from build123d import *

# Parameters (mm, degrees)
MODEL_W             = 6
MODEL_H             = 6
BOSS_EXTRUDE1_DEPTH = 6


with BuildPart() as part:
    # Model → Boss-Extrude1 (new body)
    with BuildSketch(Plane.XY):
        with BuildLine():
            Line((3491.847275697, 1193.017146611), (3491.847275697, 1187.017146611))
            Line((3491.847275697, 1187.017146611), (3485.847275697, 1187.017146611))
            Line((3485.847275697, 1187.017146611), (3485.847275697, 1193.017146611))
            Line((3485.847275697, 1193.017146611), (3474.204418554, 1193.017146611))
            ThreePointArc((3474.204418554, 1193.017146611), (3501.847275697, 1220.660003754), (3529.49013284, 1193.017146611))
            Line((3529.49013284, 1193.017146611), (3491.847275697, 1193.017146611))
        make_face()
        with Locations((3514.847275697, 1206.017146611)):
            Rectangle(MODEL_W, MODEL_H, mode=Mode.SUBTRACT)
        with Locations((3488.847275697, 1206.017146611)):
            Rectangle(MODEL_W, MODEL_H, mode=Mode.SUBTRACT)
        with Locations((3501.847275697, 1212.017146611)):
            Rectangle(MODEL_W, MODEL_H, mode=Mode.SUBTRACT)
        with Locations((3501.847275697, 1199.841605445)):
            Rectangle(MODEL_W, MODEL_H, mode=Mode.SUBTRACT)
    extrude(amount=BOSS_EXTRUDE1_DEPTH)


solid = part.part
Model file for the job. Use its own axes, mm. A direction names the side the tool comes from. Give positions to 0.01 mm unless a question says otherwise; leave off trailing zeros. Loops run counter-clockwise (first coordinate to the right, second up) from the corner with the lowest first, then second, coordinate; pieces in that order, holes last.
1) Wall check: line 1 (Y direction, x = 3502.5, z = 5.2); line 2 (Y direction, x = 3502, z = 4.2); line 3 (X direction, y = 1205, z = 3.8). Give the ranges that are in metal, low to high.
2) Saw through at A-A (z = 1). Write the cut outline in (x, y), plus the area to 3 significant figures.
3) Saw through at D-D (x = 3516.5). Write the cut outline in (y, z).
4) Flat gauge pins, fed straight in: pin 1 Ø3 at (y, z) = (1204.5, 2.5) entering from -X; pin 2 Ø3 at (x, z) = (3488.5, 4.5) entering from +Y; pin 3 Ø1.8 at (x, z) = (3515.5, 2) entering from -Y. Where does each tip first touch, or does it go through?
5) Pull direction Y, two halves, no side cores. Call faces 5 (the flat face through (3491.847, 1190, 3)), 6 (the flat face through (3504.847, 1212, 3)), 7 (the flat face through (3480, 1193.017, 3)): +Y half, -Y half, draft (parallel to the pull), parting line (faces both ways), or undercut.
6) Saw through at B-B (y = 1200). Write the cut outline in (x, z).
7) Tool access for faces 1 (the flat face through (3485.847, 1190, 3)), 2 (the flat face through (3502, 1204, 6)), 3 (the flat face through (3511, 1193.017, 3)), 4 (the flat face through (3511.847, 1206, 3)): list every direction of +Z, -Z, +X, -X, +Y, -Y with a clear straight run to the whole face (end or side of a thin tool).
8) Saw through at C-C (y = 1204). Write the cut outline in (x, z), plus the area to 3 significant figures.
Answer block:
1. line 1: y = 1193.02 to 1196.84, 1202.84 to 1209.02, 1215.02 to 1220.65
1. line 2: y = 1193.02 to 1196.84, 1202.84 to 1209.02, 1215.02 to 1220.66
1. line 3: x = 3476.94 to 3485.85, 3491.85 to 3511.85, 3517.85 to 3526.76
2. outline: (3474.2, 1193.02) - (3485.85, 1193.02) - (3485.85, 1187.02) - (3491.85, 1187.02) - (3491.85, 1193.02) - (3529.49, 1193.02) arc R27.64 ccw to start; hole (3485.85, 1203.02) - (3491.85, 1203.02) - (3491.85, 1209.02) - (3485.85, 1209.02) - close; hole (3498.85, 1196.84) - (3504.85, 1196.84) - (3504.85, 1202.84) - (3498.85, 1202.84) - close; hole (3498.85, 1209.02) - (3504.85, 1209.02) - (3504.85, 1215.02) - (3498.85, 1215.02) - close; hole (3511.85, 1203.02) - (3517.85, 1203.02) - (3517.85, 1209.02) - (3511.85, 1209.02) - close
2. area: 1,090 mm2
3. outline: (1193.02, 0) - (1203.02, 0) - (1203.02, 6) - (1193.02, 6) - close; (1209.02, 0) - (1216.46, 0) - (1216.46, 6) - (1209.02, 6) - close
4. pin 1: stops at x = 3476.07
4. pin 2: stops at y = 1217.99
4. pin 3: stops at y = 1193.02
5. face 5: draft
5. face 6: undercut
5. face 7: -Y half
6. outline: (3475.1, 0) - (3498.85, 0) - (3498.85, 6) - (3475.1, 6) - close; (3504.85, 0) - (3528.59, 0) - (3528.59, 6) - (3504.85, 6) - close
7. face 1: +Z, -Z, -X, -Y
7. face 2: +Z, +X, -X, +Y, -Y
7. face 3: +Z, -Z, +X, -Y
7. face 4: +Z, -Z
8. outline: (3476.48, 0) - (3485.85, 0) - (3485.85, 6) - (3476.48, 6) - close; (3491.85, 0) - (3511.85, 0) - (3511.85, 6) - (3491.85, 6) - close; (3517.85, 0) - (3527.21, 0) - (3527.21, 6) - (3517.85, 6) - close
8. area: 232 mm2
